```python
from build123d import *

# Parameters (mm, degrees)
F0_W      = 180
F0_H      = 190
F1_DEPTH  = 3
F2_W      = 6
F2_H      = 6
F3_DEPTH  = 3.001
F4_W      = 168
F4_H      = 25
F5_DEPTH  = 3.001
F6_DEPTH  = 1
F7_DEPTH  = 1
F8_DEPTH  = 1
F9_W      = 168
F9_H      = 134.1867442131
F10_DEPTH = 1


with BuildPart() as f1:
    # F0 (on Top) → F1 (new body)
    with BuildSketch(Plane.XY):
        with Locations((90, -95)):
            Rectangle(F0_W, F0_H)
    extrude(amount=F1_DEPTH)

    # F2 (on face) → F3 (cut, through all)
    with BuildSketch(Plane.XY.offset(3)):
        with Locations((3, -187)):
            Rectangle(F2_W, F2_H)
        with Locations((177, -187)):
            Rectangle(F2_W, F2_H)
        with Locations((177, -3)):
            Rectangle(F2_W, F2_H)
        with Locations((3, -3)):
            Rectangle(F2_W, F2_H)
    extrude(amount=-F3_DEPTH, mode=Mode.SUBTRACT)

    # F4 (on face) → F5 (cut, through all)
    with BuildSketch(Plane.XY.offset(3)):
        Polygon((6, -152.5), (6, -176.5), (12, -176.5), (12, -184), (168, -184), (168, -176.5), (174, -176.5), (174, -152.5), align=None)
        with Locations((90, -137)):
            Rectangle(F4_W, F4_H)
        with Locations((90, -109)):
            Rectangle(F4_W, F4_H)
        with Locations((90, -81)):
            Rectangle(F4_W, F4_H)
        with Locations((90, -53)):
            Rectangle(F4_W, F4_H)
        Polygon((6, -13.5), (6, -37.5), (174, -37.5), (174, -13.5), (167.9999051407, -13.5), (168, -6.0000000006), (12, -6), (11.9999051407, -13.5), align=None)
    extrude(amount=-F5_DEPTH, mode=Mode.SUBTRACT)

    # F6 (add): a face of the model
    f6_faces = [f1.faces().sort_by_distance(p)[0] for p in [
        (90, -190, 1.5),
    ]]
    extrude(f6_faces, amount=F6_DEPTH)

    # F7 (add): a face of the model
    f7_faces = [f1.faces().sort_by_distance(p)[0] for p in [
        (90, 0, 1.5),
    ]]
    extrude(f7_faces, amount=F7_DEPTH)

    # F8 (add): faces of the model
    f8_faces = [f1.faces().sort_by_distance(p)[0] for p in [
        (177, -6, 1.5),
        (3, -6, 1.5),
        (3, -184, 1.5),
        (177, -184, 1.5),
    ]]
    extrude(f8_faces, amount=F8_DEPTH, dir=(0, 1, 0))

    # F9 (on face) → F10 (cut)
    with BuildSketch(Plane(origin=(0, 0, 0), x_dir=(1, 0, 0), z_dir=(0, 0, -1))):
        with Locations((90, 92.5933721066)):
            Rectangle(F9_W, F9_H)
    extrude(amount=-F10_DEPTH, mode=Mode.SUBTRACT)


solid = f1.part
```
Design review of the part built by this model. Coordinates are the model's own, in mm. Round coordinates to 2 decimals unless told otherwise and drop trailing zeros. Write each loop counter-clockwise with the first axis right and the second up, starting at its lowest first coordinate (ties: lowest second). Pieces come first, ordered by that corner, then holes. Notation, with made-up numbers: (85, 38.25) -> (143, 38.25) arc R22 ccw to (143, 64.25) -> close; hole circle Ø9 at (47, 75). An arc over 180 degrees is marked (long way). Answer in a Markdown table with one row per item.
Q1. Clearance check with a flat-ended pin moving along its axis: pin 1 Ø2.5 at (x, y) = (73.5, -151.5) entering from -Z. State where the tip first meets the part, or that it passes through.
The answers:
| item | result |
|---|---|
| pin 1 | z = 1 |
Q2. Take a section at B-B, the plane x = 37. State the section outline as (y, z) points.
The answers:
| item | result |
|---|---|
| outline | (-191, 0) -> (-184, 0) -> (-184, 3) -> (-191, 3) -> close; (-152.5, 1) -> (-149.5, 1) -> (-149.5, 3) -> (-152.5, 3) -> close; (-124.5, 1) -> (-121.5, 1) -> (-121.5, 3) -> (-124.5, 3) -> close; (-96.5, 1) -> (-93.5, 1) -> (-93.5, 3) -> (-96.5, 3) -> close; (-68.5, 1) -> (-65.5, 1) -> (-65.5, 3) -> (-68.5, 3) -> close; (-40.5, 1) -> (-37.5, 1) -> (-37.5, 3) -> (-40.5, 3) -> close; (-6, 0) -> (1, 0) -> (1, 3) -> (-6, 3) -> close |
Q3. To check wall thickness, follow L1, parallel to X at y = -132.5, z = 1.6; L2, parallel to X at y = -11.5, z = 0.6; L3, parallel to Y at x = 29, z = 0.6. State the ranges of each line that lie inside material, in increasing order. Write a range as [from, to].
The answers:
| item | result |
|---|---|
| L1 | [0, 6], [174, 180] |
| L2 | [0, 12], [168, 180] |
| L3 | [-191, -184], [-6, 1] |
Q4. Take a section at A-A, the plane y = -99. State the section outline as (x, z) points.
The answers:
| item | result |
|---|---|
| outline | (0, 0) -> (6, 0) -> (6, 3) -> (0, 3) -> close; (174, 0) -> (180, 0) -> (180, 3) -> (174, 3) -> close |
Q5. Take a section at C-C, the plane z = 1.6. Count the separate pieces of the cut face and the enclosed holes in it, then the cut area to 3 significant figures.
The answers:
| item | result |
|---|---|
| separate pieces | 1 |
| enclosed holes | 6 |
| area | 7,200 mm² |
